The model under review builds one solid part; all positions refer to its coordinate system, in mm. A direction names the side the tool comes from. Coordinates: 2 decimals unless noted, no trailing zeros. Write each loop counter-clockwise with the first axis right and the second up, starting at its lowest first coordinate (ties: lowest second). Pieces come first, ordered by that corner, then holes.
1) For P1, Ø4, axis at x = 2.5, y = -2.5, coming from the -Z side, flat-tipped, find the tip position at first contact; note if it passes through.
2) For line 1 (X direction, y = 2.75, z = 2.6); line 2 (X direction, y = -0.75, z = 0.9); line 3 (X direction, y = -1, z = 2.3), list the stretches that pass through material, from the lowest coordinate up.
3) Add section D-D, the plane z = 1.35. State the section outline as (x, y) points.
4) Machinability: for faces 4 (the flat face through (-10.323, 4, 1)), 5 (the cylindrical face through (-16.222, -5.842, 1.479)), which of the approach directions +Z, -Z, +X, -X, +Y, -Y give a long, thin tool a straight path to every point of the face, cutting with its end or side? Answer none if there is none.
5) Add section A-A, the plane y = 4.5. State the section outline as (x, z) points, then the cut area to 3 significant figures.
6) Mouldability with a two-part tool opening along Y and no side actions: class faces 1 (the cylindrical face through (0.68, 0.15, 1.48)), 2 (the flat face through (6.177, 1, 1)), 3 (the cylindrical face through (5.607, -5.81, 1.479)) as released by +Y, released by -Y, zero draft, split by the parting line, or undercut.
7) Add section B-B, the plane x = -13.5. State the section outline as (y, z) points.
8) Add section C-C, the plane y = -0.75. State the section outline as (x, z) points.
from build123d import *

# Parameters (mm, degrees)
SKETCH1_R           = 1.5
BOSS_EXTRUDE1_DEPTH = 3


with BuildPart() as part:
    # Sketch1 → Boss-Extrude1 (new body)
    with BuildSketch(Plane.XY):
        with BuildLine():
            Line((-10.322941477, 5.588109805), (-10.322941477, 2.588109805))
            Line((-10.322941477, 2.588109805), (-0.322941477, 2.588109805))
            Line((-0.322941477, 2.588109805), (-0.322941477, 5.588109805))
            Line((-0.322941477, 5.588109805), (6.177058523, 5.588109805))
            Line((6.177058523, 5.588109805), (6.177058523, -4.411890195))
            ThreePointArc((6.177058523, -4.411890195), (5.591272086, -5.826103757), (4.177058523, -6.411890195))
            Line((4.177058523, -6.411890195), (-14.822941477, -6.411890195))
            ThreePointArc((-14.822941477, -6.411890195), (-16.237155039, -5.826103757), (-16.822941477, -4.411890195))
            Line((-16.822941477, -4.411890195), (-16.822941477, 5.588109805))
            Line((-16.822941477, 5.588109805), (-10.322941477, 5.588109805))
        make_face()
        with Locations((-12.822941477, 0.088109805)):
            Circle(SKETCH1_R, mode=Mode.SUBTRACT)
        with Locations((2.177058523, 0.088109805)):
            Circle(SKETCH1_R, mode=Mode.SUBTRACT)
    extrude(amount=BOSS_EXTRUDE1_DEPTH)


solid = part.part
Geometry results:
1. P1: stops at z = 0
2. line 1: x = -16.82 to -10.32, -0.32 to 6.18
2. line 2: x = -16.82 to -14.07, -11.58 to 0.93, 3.42 to 6.18
2. line 3: x = -16.82 to -13.86, -11.79 to 1.14, 3.21 to 6.18
3. outline: (-16.82, -4.41) arc R2 ccw to (-14.82, -6.41) - (4.18, -6.41) arc R2 ccw to (6.18, -4.41) - (6.18, 5.59) - (-0.32, 5.59) - (-0.32, 2.59) - (-10.32, 2.59) - (-10.32, 5.59) - (-16.82, 5.59) - close; hole circle Ø3 at (-12.82, 0.09); hole circle Ø3 at (2.18, 0.09)
4. face 4: +Z, -Z, +Y
4. face 5: +Z, -Z, -X, -Y
5. outline: (-16.82, 0) - (-10.32, 0) - (-10.32, 3) - (-16.82, 3) - close; (-0.32, 0) - (6.18, 0) - (6.18, 3) - (-0.32, 3) - close
5. area: 39.0 mm2
6. face 1: undercut
6. face 2: zero draft
6. face 3: released by -Y
7. outline: (-6.41, 0) - (-1.25, 0) - (-1.25, 3) - (-6.41, 3) - close; (1.43, 0) - (5.59, 0) - (5.59, 3) - (1.43, 3) - close
8. outline: (-16.82, 0) - (-14.07, 0) - (-14.07, 3) - (-16.82, 3) - close; (-11.58, 0) - (0.93, 0) - (0.93, 3) - (-11.58, 3) - close; (3.42, 0) - (6.18, 0) - (6.18, 3) - (3.42, 3) - close
